from build123d import *

# Parameters (mm, degrees)
F0_W     = 38.277834
F0_H     = 285.75
F1_DEPTH = 1879.6
F2_SIZE  = 38.1
F3_W     = 1841.5
F3_H     = 19.05
F4_DEPTH = 19.05


with BuildPart() as f1:
    # F0 (on Front) → F1 (new body)
    with BuildSketch(Plane.XZ):
        Rectangle(F0_W, F0_H)
    extrude(amount=F1_DEPTH)

    # F2
    f2_edges = [f1.edges().sort_by_distance(p)[0] for p in [
        (19.138917, -1879.6, 0),
        (19.138917, 0, 0),
    ]]
    chamfer(f2_edges, length=F2_SIZE)

    # F3 (on face) → F4 (cut)
    with BuildSketch(Plane.YZ.offset(19.138917)):
        with Locations((-939.8, 133.35)):
            Rectangle(F3_W, F3_H)
    extrude(amount=-F4_DEPTH, mode=Mode.SUBTRACT)


solid = f1.part
Here's how the part is built. I have some questions about the finished solid (model axes, mm). Coordinates: 2 decimals unless noted, no trailing zeros. Write each loop counter-clockwise with the first axis right and the second up, starting at its lowest first coordinate (ties: lowest second). Pieces come first, ordered by that corner, then holes.
1) I'm going to push flat-ended pins straight in: pin 1 (4 mm diameter, centred on x = -11.5, z = -10.5, fed in from +Y); pin 2 (12 mm diameter, centred on x = -12, z = -78, fed in from -Y); pin 3 (1.5 mm diameter, centred on x = -0.5, z = -25, fed in from +Y). Where does each tip first touch, or does it pass through?
Filled in:
pin 1: stops at y = -5.46
pin 2: stops at y = -1878.64
pin 3: stops at y = -17.71
2) If I drill on line 1 (Z direction, x = 4, y = -117) (3 decimals); line 2 (Y direction, x = 15.5, z = -113.5); line 3 (Y direction, x = 7, z = 117), over which ranges is the centre line in solid material (lowest first)?
Filled in:
line 1: z = -142.875 to 123.825
line 2: y = -1845.14 to -34.46
line 3: y = -1853.64 to -25.96
3) If we section it at A-A (z = 43.5): List the corners of the cut face in (x, y) for me.
Filled in:
outline: (-19.14, -1879.6) - (-18.96, -1879.6) - (19.14, -1841.5) - (19.14, -38.1) - (-18.96, 0) - (-19.14, 0) - close
4) If we section it at C-C (x = 8.5): List the corners of the cut face in (y, z) for me (3 decimals).
Filled in:
outline: (-1852.139, -142.875) - (-27.461, -142.875) - (-27.461, 123.825) - (-1852.139, 123.825) - close
5) If we section it at B-B (y = -848): List the corners of the cut face in (x, z) for me (3 decimals).
Filled in:
outline: (-19.139, -142.875) - (19.139, -142.875) - (19.139, 123.825) - (0.089, 123.825) - (0.089, 142.875) - (-19.139, 142.875) - close
